from build123d import *

# Parameters (mm, degrees)
BOSS_EXTRUDE1_DEPTH = 50
SKETCH2_W           = 19
SKETCH2_H           = 50
CUT_EXTRUDE1_DEPTH  = 38
SKETCH3_W           = 25
SKETCH3_H           = 36
CUT_EXTRUDE2_DEPTH  = 38


with BuildPart() as part:
    # Sketch1 → Boss-Extrude1 (new, symmetric)
    with BuildSketch(Plane(origin=(0, 0, 0), x_dir=(-1, 0, 0), z_dir=(0, 1, 0))):
        Polygon((0, 0), (12, 0), (12, 6), (51, 6), (51, 0), (63, 0), (63, 75), (25, 75), (25, 25), (0, 25), align=None)
    extrude(amount=BOSS_EXTRUDE1_DEPTH, both=True)

    # Sketch2 → Cut-Extrude1 (cut)
    with BuildSketch(Plane.XY.offset(75)):
        with Locations((-34.5, 0)):
            Rectangle(SKETCH2_W, SKETCH2_H)
    extrude(amount=-CUT_EXTRUDE1_DEPTH, mode=Mode.SUBTRACT)

    # Sketch3 → Cut-Extrude2 (cut)
    with BuildSketch(Plane.XY.offset(25)):
        with Locations((-12.5, 0)):
            Rectangle(SKETCH3_W, SKETCH3_H)
    extrude(amount=-CUT_EXTRUDE2_DEPTH, mode=Mode.SUBTRACT)


solid = part.part
Build history of the part. All positions in model axes, mm. A direction names the side the tool comes from. Coordinates: 2 decimals unless noted, no trailing zeros. Order: outer loops, then holes, each group sorted by start corner. A loop starts at its lowest first (then second) coordinate and runs counter-clockwise, first axis right, second up. Notation, with made-up numbers: (54, 67) -> (66, 67) arc R29 cw to (66, 103) -> close; hole circle Ø7 at (65.25, 38). An arc over 180 degrees is marked (long way). One line per item, written item: value.
(1) Probe line 1 (Y direction, x = -20, z = 16.5); line 2 (Y direction, x = -40.5, z = 43.5); line 3 (Z direction, x = -44, y = 34). List the from-to ranges inside material, lowest first. Write a range as [from, to].
Checked values:
line 1: [-50, -18], [18, 50]
line 2: [-50, -25], [25, 50]
line 3: [6, 75]
(2) Slice it at C-C, the plane y = 0. List the corners of the cut face in (x, z), plus the area to 3 significant figures.
Checked values:
outline: (-63, 0) -> (-51, 0) -> (-51, 6) -> (-25, 6) -> (-25, 37) -> (-44, 37) -> (-44, 75) -> (-63, 75) -> close
area: 1,970 mm2
(3) Drop flat-ended pins along their axis: pin 1 Ø5 at (y, z) = (21, 66) entering from +X; pin 2 Ø20 at (x, y) = (-9.5, 32) entering from +Z; pin 3 Ø19.5 at (x, y) = (-30, 0) entering from -Z. Give the stop position or say it passes through.
Checked values:
pin 1: x = -44
pin 2: z = 25
pin 3: z = 6
(4) Mould opens along X. For faces 4 (the flat face through (-31, 1, 6)), 5 (the flat face through (-13, -34, 25)), 6 (the flat face through (-44, 0, 56)), 7 (the flat face through (-12, -34, 3)) say: pulls with the +X half, pulls with the -X half, needs draft (parallel to the pull), parting line crosses it, or undercut.
Checked values:
face 4: undercut
face 5: needs draft
face 6: pulls with the +X half
face 7: undercut
(5) Tool access for faces 1 (the flat face through (-51, 1, 3)), 2 (the flat face through (-35, 0, 37)), 3 (the flat face through (-13, 34, 25)): list every direction of +Z, -Z, +X, -X, +Y, -Y with a clear straight run to the whole face (end or side of a thin tool).
Checked values:
face 1: -Z, +Y, -Y
face 2: +Z, +X
face 3: +Z, +X, +Y, -Y
(6) Slice it at D-D, the plane y = -20. List the corners of the cut face in (x, z), plus the area to 3 significant figures.
Checked values:
outline: (-63, 0) -> (-51, 0) -> (-51, 6) -> (-12, 6) -> (-12, 0) -> (0, 0) -> (0, 25) -> (-25, 25) -> (-25, 37) -> (-44, 37) -> (-44, 75) -> (-63, 75) -> close
area: 2,520 mm2
(7) Slice it at A-A, the plane x = -21. List the corners of the cut face in (y, z), plus the area to 3 significant figures.
Checked values:
outline: (-50, 6) -> (-18, 6) -> (-18, 25) -> (-50, 25) -> close; (18, 6) -> (50, 6) -> (50, 25) -> (18, 25) -> close
area: 1,220 mm2
(8) Slice it at B-B, the plane z = 10. List the corners of the cut face in (x, y).
Checked values:
outline: (-63, -50) -> (0, -50) -> (0, -18) -> (-25, -18) -> (-25, 18) -> (0, 18) -> (0, 50) -> (-63, 50) -> close
